Work out the finished part from the listing and answer in its coordinate system (mm). Face numbers are marked on the shaded views. A direction names the side the tool comes from. Coordinates: 2 decimals unless noted, no trailing zeros. Loops run counter-clockwise (first coordinate to the right, second up) from the corner with the lowest first, then second, coordinate; pieces in that order, holes last. Notation, with made-up numbers: (-13, 5) - (37, 5) arc R20 ccw to (37, 26) - close; hole circle Ø8 at (66, 43.5). An arc over 180 degrees is marked (long way). Write each question's results on one line, items separated by ' | '. Start each with the question number.
1. A cutting plane is placed at C-C on z = -5.5. Determine the outline of the cut face in (x, y).
2. Each of these flat-tipped pins is pushed along its axis until it touches: P1, Ø3, axis at x = -12.99, y = 7.5, coming from the -Z side; P2, Ø10, axis at x = 17.5, z = -0.5, coming from the +Y side; P3, Ø1.5, axis at y = 6.5, z = 3.5, coming from the -X side; P4, Ø2, axis at x = 0, y = 15, coming from the -Z side. Where does it stop, or does it pass through?
3. A cutting plane is placed at A-A on x = 0. Determine the outline of the cut face in (y, z).
4. A cutting plane is placed at D-D on x = 8.5. Determine the outline of the cut face in (y, z), then the cut area to 3 significant figures.
5. Which of the six approach directions +Z, -Z, +X, -X, +Y, -Y give full straight-line access (tool end or side, diameter ignored) to the marked faces 4, 5 and 6?
6. A cutting plane is placed at B-B on y = -7.5. Determine the outline of the cut face in (x, z), then the cut area to 3 significant figures.
7. Determine the mould class of the marked faces 1, 2 and 3 for opening direction X: released by +X, released by -X, zero draft, split by the parting line, or undercut.
8. Find the intervals of material crossed by line 1 along Y through (x, z) = (0, 2.5); line 2 along Z through (x, y) = (19, -5); line 3 along Z through (x, y) = (6, 1.5), in increasing order. Write a range as [from, to].
from build123d import *

# Parameters (mm, degrees)
SKETCH_2_R          = 29.5
EXTRUDE_1_DEPTH     = 2
SKETCH_3_R          = 25
EXTRUDE_2_DEPTH     = 10
SKETCH_4_R          = 5.1
EXTRUDE_3_DEPTH     = 8.2
SKETCH_7_R          = 1.4
CUT_EXTRUDE_3_DEPTH = 12
CUT_EXTRUDE_4_REACH = 45.411
SKETCH_9_R          = 6.5
EXTRUDE_START       = -5.9
SKETCH_10_R         = 6.5
SKETCH_10_R_2       = 5.5
EXTRUDE_4_DEPTH     = 5.9


with BuildPart() as part:
    # 草图2 → 凸台-拉伸1 (new body)
    with BuildSketch(Plane.XY):
        Circle(SKETCH_2_R)
    extrude(amount=EXTRUDE_1_DEPTH)

    # 草图3 → 凸台-拉伸2 (add)
    with BuildSketch(Plane.XY.offset(2)):
        Circle(SKETCH_3_R)
    extrude(amount=EXTRUDE_2_DEPTH)

    # 草图4 → 凸台-拉伸3 (add)
    with BuildSketch(Plane(origin=(0, 0, 0), x_dir=(-1, 0, 0), z_dir=(0, 0, -1))):
        with Locations(Location((17, 0, 0), (0, 0, 180))):
            Circle(SKETCH_4_R)
        with Locations(Location((8.5, -14.722431864, 0), (0, 0, 180))):
            Circle(SKETCH_4_R)
        with Locations(Location((-8.5, -14.722431864, 0), (0, 0, 180))):
            Circle(SKETCH_4_R)
        with Locations(Location((-17, 0, 0), (0, 0, 180))):
            Circle(SKETCH_4_R)
        with Locations(Location((-8.5, 14.722431864, 0), (0, 0, 180))):
            Circle(SKETCH_4_R)
        with Locations(Location((8.5, 14.722431864, 0), (0, 0, 180))):
            Circle(SKETCH_4_R)
    extrude(amount=EXTRUDE_3_DEPTH)

    # 草图7 → 切除-拉伸3 (cut)
    with BuildSketch(Plane.XY.offset(12)):
        with Locations((12.990381057, 7.5)):
            Circle(SKETCH_7_R)
        with Locations((12.990381057, -7.5)):
            Circle(SKETCH_7_R)
        with Locations((0, -15)):
            Circle(SKETCH_7_R)
        with Locations((-12.990381057, -7.5)):
            Circle(SKETCH_7_R)
        with Locations((-12.990381057, 7.5)):
            Circle(SKETCH_7_R)
        with Locations((0, 15)):
            Circle(SKETCH_7_R)
    extrude(amount=-CUT_EXTRUDE_3_DEPTH, mode=Mode.SUBTRACT)

    # 草图9 → 切除-拉伸4 (cut, up to next)
    with BuildSketch(Plane(origin=(0, 0, 0), x_dir=(-1, 0, 0), z_dir=(0, 0, -1)), mode=Mode.PRIVATE) as cut_extrude_4_sk1:
        Circle(SKETCH_9_R)
    cut_extrude_4_tool1 = extrude(cut_extrude_4_sk1.sketch, amount=-CUT_EXTRUDE_4_REACH, mode=Mode.PRIVATE) & part.part
    add(cut_extrude_4_tool1.solids().sort_by_distance((0, 0, 0))[0], mode=Mode.SUBTRACT)

    # 草图10 → 凸台-拉伸4 (add)
    with BuildSketch(Plane.XY.offset(12).offset(EXTRUDE_START)):
        with Locations(Location((0, 0, 0), (0, 0, 180))):
            Circle(SKETCH_10_R)
        Circle(SKETCH_10_R_2, mode=Mode.SUBTRACT)
    extrude(amount=EXTRUDE_4_DEPTH)


solid = part.part
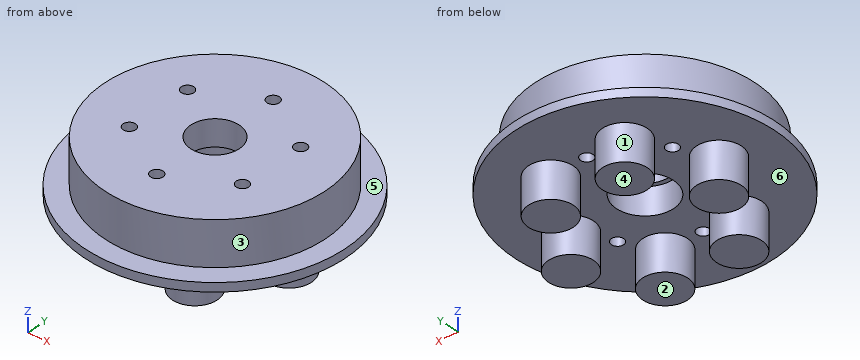
Values:
1) outline: circle Ø10.2 at (-17, 0); circle Ø10.2 at (-8.5, -14.72); circle Ø10.2 at (-8.5, 14.72); circle Ø10.2 at (8.5, -14.72); circle Ø10.2 at (8.5, 14.72); circle Ø10.2 at (17, 0)
2) P1: z = 0 | P2: y = 26.71 | P3: x = -24.33 | P4: through
3) outline: (-29.5, 0) - (-16.4, 0) - (-16.4, 12) - (-25, 12) - (-25, 2) - (-29.5, 2) - close; (-13.6, 0) - (-6.5, 0) - (-6.5, 6.1) - (-5.5, 6.1) - (-5.5, 12) - (-13.6, 12) - close; (5.5, 6.1) - (6.5, 6.1) - (6.5, 0) - (13.6, 0) - (13.6, 12) - (5.5, 12) - close; (16.4, 0) - (29.5, 0) - (29.5, 2) - (25, 2) - (25, 12) - (16.4, 12) - close
4) outline: (-28.25, 0) - (-19.82, 0) - (-19.82, -8.2) - (-9.62, -8.2) - (-9.62, 0) - (9.62, 0) - (9.62, -8.2) - (19.82, -8.2) - (19.82, 0) - (28.25, 0) - (28.25, 2) - (23.51, 2) - (23.51, 12) - (-23.51, 12) - (-23.51, 2) - (-28.25, 2) - close | area: 750 mm^2
5) face 4: -Z, +X, -X, +Y, -Y | face 5: +Z | face 6: -Z
6) outline: (-28.53, 0) - (-14.39, 0) - (-14.39, 12) - (-23.85, 12) - (-23.85, 2) - (-28.53, 2) - close; (-11.59, 0) - (11.59, 0) - (11.59, 12) - (-11.59, 12) - close; (14.39, 0) - (28.53, 0) - (28.53, 2) - (23.85, 2) - (23.85, 12) - (14.39, 12) - close | area: 524 mm^2
7) face 1: undercut | face 2: zero draft | face 3: split by the parting line
8) line 1: [-25, -16.4], [-13.6, -6.5], [6.5, 13.6], [16.4, 25] | line 2: [0, 12] | line 3: [6.1, 12]
